For this review, take the finished solid that the model builds, in its own axes (mm). A direction names the side the tool comes from. Round coordinates to 2 decimals unless told otherwise and drop trailing zeros. Loops run counter-clockwise (first coordinate to the right, second up) from the corner with the lowest first, then second, coordinate; pieces in that order, holes last. Notation, with made-up numbers: (73.5, -16) -> (81.5, -16) arc R23 cw to (81.5, 6) -> close; hole circle Ø8 at (16, 81.25). An arc over 180 degrees is marked (long way). Write each question's results on one line, items separated by ' | '.
```python
from build123d import *


with BuildPart() as part:
    # Sketch1 → Revolve1 (revolve)
    with BuildSketch(Plane.XY):
        Polygon((-6.35, -13.081), (-6.35, -64.29375), (-7.14375, -64.29375), (-7.14375, -51.59375), (-9.525, -49.2125), (-9.525, -25.4), (-19.05, -25.4), (-19.05, -19.431), (-16.51, -19.431), (-16.51, -15.875), (-19.05, -15.875), (-19.05, -13.081), (-16.51, -13.081), (-16.51, -9.525), (-19.05, -9.525), (-19.05, 0), (-6.35, 0), (-6.35, -3.175), (-8.89, -3.175), (-8.89, -6.731), (-6.35, -6.731), (-6.35, -9.525), (-8.89, -9.525), (-8.89, -13.081), align=None)
    revolve(axis=Axis((0, 0, 0), (0, -1, 0)))


solid = part.part
```
1. Consider section B-B (x = -15). State the section outline as (y, z) points (3 decimals).
Values found:
outline: (-25.4, -11.743) -> (-19.431, -11.743) -> (-19.431, -6.898) -> (-15.875, -6.898) -> (-15.875, -11.743) -> (-13.081, -11.743) -> (-13.081, -6.898) -> (-9.525, -6.898) -> (-9.525, -11.743) -> (0, -11.743) -> (0, 11.743) -> (-9.525, 11.743) -> (-9.525, 6.898) -> (-13.081, 6.898) -> (-13.081, 11.743) -> (-15.875, 11.743) -> (-15.875, 6.898) -> (-19.431, 6.898) -> (-19.431, 11.743) -> (-25.4, 11.743) -> close
2. For pin 1 (10.5 mm diameter, centred on x = 0, z = 0, fed in from -Y); pin 2 (1.5 mm diameter, centred on y = -42, z = 8, fed in from +X); pin 3 (12 mm diameter, centred on y = -7, z = -8.5, fed in from +X); pin 4 (3 mm diameter, centred on x = 10.5, y = -15.5, fed in from +Z), all flat-tipped, find the tip position at first contact; note any pin that passes through.
Values found:
pin 1: passes through | pin 2: stops at x = 6.18 | pin 3: stops at x = 18.89 | pin 4: stops at z = 16.79
3. Consider section C-C (y = -54.5). State the section outline as (x, z) points.
Values found:
outline: circle Ø14.29 at (0, 0); hole circle Ø12.7 at (0, 0)
4. Draft analysis for pull direction Y (two halves, no side actions). For faces 1 (the face through (4, -9.525, 6)), 2 (the face through (-6, -64.294, 3)), 3 (the face through (5, 0, -5)), state which applies: released by +Y, released by -Y, zero draft, split by the parting line, or undercut.
Values found:
face 1: undercut | face 2: released by -Y | face 3: released by +Y
5. Consider section A-A (y = -33.5). State the section outline as (x, z) points (3 decimals).
Values found:
outline: circle Ø19.05 at (0, 0); hole circle Ø12.7 at (0, 0)
6. Tool access review of faces 4 (the face through (15.12, -14.46, 11.59)), 5 (the face through (7.137, -57.855, -0.314)), 6 (the face through (6, -13.081, -16)): name each direction out of +Z, -Z, +X, -X, +Y, -Y from which nothing blocks a thin tool from reaching the whole face with its end or side.
Values found:
face 4: +Y, -Y | face 5: -Y | face 6: none
7. To check wall thickness, follow probe 1 along Y at (x, z) = (17.5, 1.5) (3 decimals); probe 2 along Z at (x, y) = (0, -25); probe 3 along X at (y, z) = (-47, 0) (3 decimals). State the ranges of each line that lie inside material, in increasing order.
Values found:
probe 1: y = -25.4 to -19.431, -15.875 to -13.081, -9.525 to 0 | probe 2: z = -19.05 to -6.35, 6.35 to 19.05 | probe 3: x = -9.525 to -6.35, 6.35 to 9.525
